Answer from the drawing. Dimensions are ordinates in mm from the lowest x, y and z of the part. Give positions to 0.01 mm unless a question says otherwise; leave off trailing zeros. Loops run counter-clockwise (first coordinate to the right, second up) from the corner with the lowest first, then second, coordinate; pieces in that order, holes last. Notation, with made-up numbers: (-25.5, -39) - (17.5, -39) arc R18 cw to (17.5, -18) - close; hole circle Ø3 at (5, 5). An arc over 180 degrees is marked (long way). Write each question's results on one line, items separated by ' | '. Start each with the question number.
Q1. Given pin 1 (12 mm diameter, centred on x = 10.5, y = 8.5, fed in from +Z) (1 decimal); pin 2 (6 mm diameter, centred on x = 3.5, z = 37.5, fed in from -Y); pin 3 (8 mm diameter, centred on x = 17.5, z = 40, fed in from -Y), each flat-ended and moving along its own axis, determine where each tip first touches the part or whether it passes through.
Q2. The part is cut by section B-B, the plane z = 57.5. Write down the section's boundary in (x, y), plus the area to 3 significant figures.
Q3. Find the intervals of material crossed by line 1 (Z direction, x = 5.5, y = 26.5) (1 decimal); line 2 (Z direction, x = 4, y = 3) (1 decimal); line 3 (Y direction, x = 3.25, z = 30) (1 decimal), in increasing order. Write a range as from..to.
Q4. The part is cut by section C-C, the plane y = 20.5. Write down the section's boundary in (x, z).
Q5. The part is cut by section A-A, the plane x = 3.25. Write down the section's boundary in (y, z) (1 decimal).
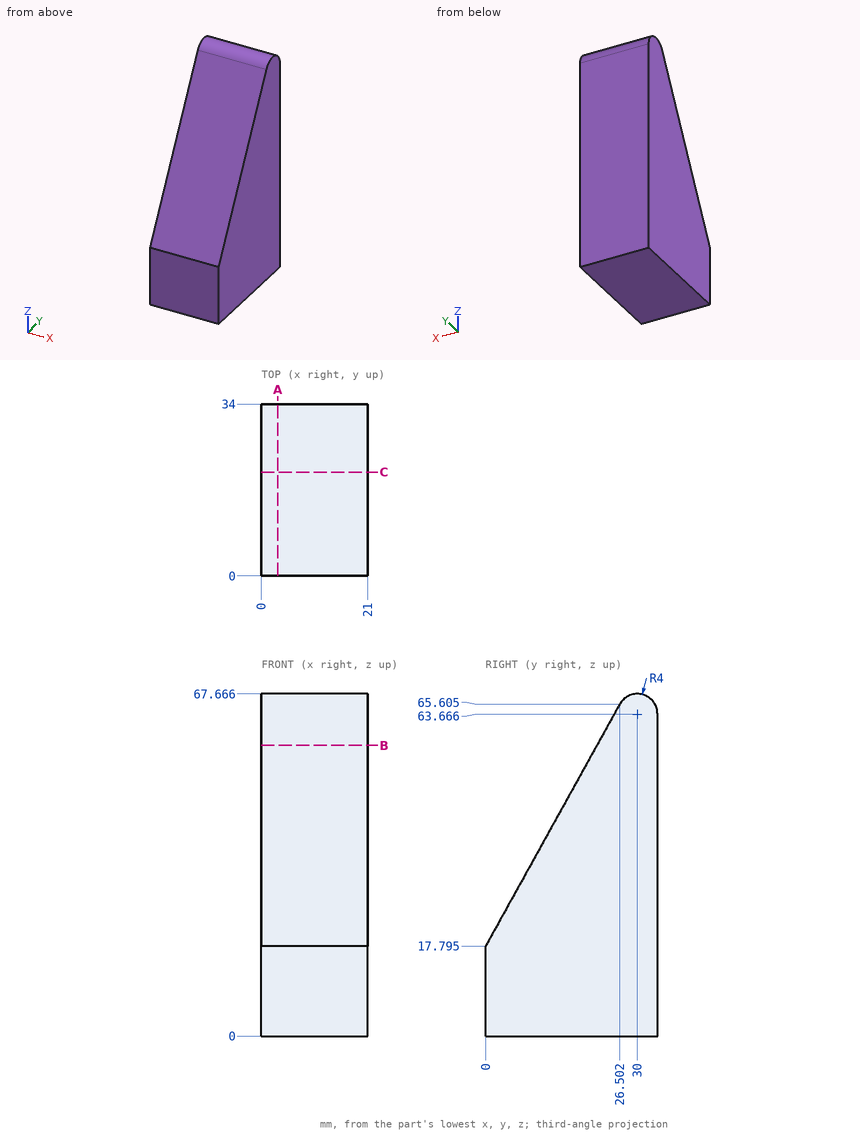
Check sheet entries:
1) pin 1: stops at z = 44 | pin 2: stops at y = 9.26 | pin 3: stops at y = 10.09
2) outline: (0, 22.01) - (21, 22.01) - (21, 34) - (0, 34) - close | area: 252 mm^2
3) line 1: z = 0..65.6 | line 2: z = 0..23.2 | line 3: y = 6.8..34
4) outline: (0, 0) - (21, 0) - (21, 54.78) - (0, 54.78) - close
5) outline: (0, 0) - (34, 0) - (34, 63.7) arc R4 ccw to (26.5, 65.6) - (0, 17.8) - close
